Work out the finished part from the listing and answer in its coordinate system (mm). A direction names the side the tool comes from. Round coordinates to 2 decimals unless told otherwise and drop trailing zeros. Write each loop counter-clockwise with the first axis right and the second up, starting at its lowest first coordinate (ties: lowest second). Pieces come first, ordered by that corner, then holes. Notation, with made-up numbers: (60.25, -27) - (115.25, -27) arc R31 ccw to (115.25, -1) - close; hole circle Ø7 at (-16.75, 3.25). An arc over 180 degrees is marked (long way). Answer as a JSON object with one key per item and string values.
```python
from build123d import *

# Parameters (mm, degrees)
SKETCH2_W                                       = 41.91
SKETCH2_H                                       = 56.947562
BOSS_EXTRUDE1_DEPTH                             = 7.62
CBORE_FOR_10_SOCKET_HEAD_CAP_SCREW1_D           = 5.1054
CBORE_FOR_10_SOCKET_HEAD_CAP_SCREW1_CBORE_D     = 9.525
CBORE_FOR_10_SOCKET_HEAD_CAP_SCREW1_CBORE_DEPTH = 4.826


with BuildPart() as part:
    # Sketch2 → Boss-Extrude1 (new body)
    with BuildSketch(Plane(origin=(0, 0, 0), x_dir=(1, 0, 0), z_dir=(0, 1, 0))):
        Rectangle(SKETCH2_W, SKETCH2_H)
    extrude(amount=BOSS_EXTRUDE1_DEPTH)

    # CBORE for #10 Socket Head Cap Screw1 (through all)
    with Locations(Plane(origin=(-20.955, 7.62, 28.473781), x_dir=(-1, 0, 0), z_dir=(0, 1, 0))):
        with Locations((-5.955, -10), (-35.955, -10)):
            CounterBoreHole(CBORE_FOR_10_SOCKET_HEAD_CAP_SCREW1_D / 2, CBORE_FOR_10_SOCKET_HEAD_CAP_SCREW1_CBORE_D / 2, CBORE_FOR_10_SOCKET_HEAD_CAP_SCREW1_CBORE_DEPTH)


solid = part.part
```
Item 1: Consider line 1 along Z through (x, y) = (15, 2); line 2 along Z through (x, y) = (15, 5.95); line 3 along Y through (x, z) = (-11.5, 17.5). Determine where each line is inside the solid, lowest interval first.
Results found:
{"line 1": "-28.47 to 15.92, 21.03 to 28.47", "line 2": "-28.47 to 13.71, 23.24 to 28.47", "line 3": "0 to 2.79"}
Item 2: For faces 4 (the flat face through (0, 4, -28.474)), 5 (the cylindrical face through (18.8, 5.2, 15.6)), determine the directions among +Z, -Z, +X, -X, +Y, -Y from which every point of the face is accessible in a straight line to the end or side of a thin tool.
Results found:
{"face 4": "-Z, +X, -X, +Y, -Y", "face 5": "+Y"}
Item 3: Each of these flat-tipped pins is pushed along its axis until it touches: P1, Ø6.5, axis at x = -15, z = 18.47, coming from the +Y side; P2, Ø10.5, axis at x = -13.5, z = 20, coming from the +Y side. Where does it stop, or does it pass through?
Results found:
{"P1": "y = 2.79", "P2": "y = 7.62"}
Item 4: A cutting plane is placed at B-B (y = 6). Write down the section's boundary in (x, z) (1 decimal), and give its area (3 significant figures).
Results found:
{"outline": "(-21, -28.5) - (21, -28.5) - (21, 28.5) - (-21, 28.5) - close; hole circle Ø9.5 at (-15, 18.5); hole circle Ø9.5 at (15, 18.5)", "area": "2,240 mm²"}
Item 5: A cutting plane is placed at A-A (x = 15). Write down the section's boundary in (y, z), and give its area (3 significant figures).
Results found:
{"outline": "(0, -28.47) - (7.62, -28.47) - (7.62, 13.71) - (2.79, 13.71) - (2.79, 15.92) - (0, 15.92) - close; (0, 21.03) - (2.79, 21.03) - (2.79, 23.24) - (7.62, 23.24) - (7.62, 28.47) - (0, 28.47) - close", "area": "374 mm²"}
Item 6: Determine the mould class of faces 1 (the flat face through (20.955, 4, 0)), 2 (the flat face through (0, 4, 28.474)), 3 (the flat face through (13, 2.794, 16)) for opening direction X: pulls with the +X half, pulls with the -X half, needs draft (parallel to the pull), parting line crosses it, or undercut.
Results found:
{"face 1": "pulls with the +X half", "face 2": "needs draft", "face 3": "undercut"}
